Geometry check sheet. Reference: the model listing, model coordinates, mm. Round coordinates to 2 decimals unless told otherwise and drop trailing zeros. Order: outer loops, then holes, each group sorted by start corner. A loop starts at its lowest first (then second) coordinate and runs counter-clockwise, first axis right, second up. Notation, with made-up numbers: (-10, -23) -> (5, -23) arc R30 cw to (5, 2) -> close; hole circle Ø7 at (65.25, -25.5). An arc over 180 degrees is marked (long way). Use a Markdown table: item, result. Add a question column.
Item 1: Gauge pin test, flat ends, axial feed: pin 1 Ø4.5 at (y, z) = (8, 2.23) entering from -X; pin 2 Ø6 at (y, z) = (8, 2.23) entering from -X. Record the tip position at first contact, or that the pin passes through.
Item 2: Sectioned sample at B-B, the plane y = 284.5. Record the cut outline in (x, z), and give its area (3 significant figures).
Item 3: Material ranges on probe 1 along X at (y, z) = (335.5, 6.75); probe 2 along Z at (x, y) = (3, 106); probe 3 along Y at (x, z) = (9, 2), recorded low to high. Write a range as [from, to].
Item 4: Sectioned sample at A-A, the plane x = 0.25. Record the cut outline in (y, z).
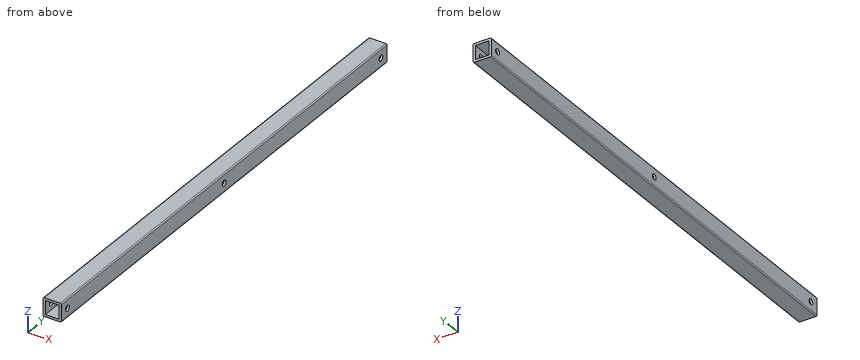
from build123d import *

# Parameters (mm, degrees)
SKETCH1_W           = 16
SKETCH1_H           = 16
SKETCH1_W_2         = 12
SKETCH1_H_2         = 12
BOSS_EXTRUDE1_DEPTH = 432
FILLET1_R           = 1
SKETCH2_R           = 2.5
CUT_EXTRUDE1_DEPTH  = 16
SKETCH3_R           = 2.5
CUT_EXTRUDE2_DEPTH  = 16


with BuildPart() as part:
    # Sketch1 → Boss-Extrude1 (new body)
    with BuildSketch(Plane(origin=(0, 0, 0), x_dir=(1, 0, 0), z_dir=(0, 1, 0))):
        with Locations((2.483870968, -2.225806452)):
            Rectangle(SKETCH1_W, SKETCH1_H)
        with Locations((2.483870968, -2.225806452)):
            Rectangle(SKETCH1_W_2, SKETCH1_H_2, mode=Mode.SUBTRACT)
    extrude(amount=BOSS_EXTRUDE1_DEPTH)

    # Fillet1
    fillet1_edges = [part.edges().sort_by_distance(p)[0] for p in [
        (-5.516129032, 216, -5.774193548),
        (10.483870968, 216, -5.774193548),
        (10.483870968, 216, 10.225806452),
        (-5.516129032, 216, 10.225806452),
    ]]
    fillet(fillet1_edges, radius=FILLET1_R)

    # Sketch2 → Cut-Extrude1 (cut)
    with BuildSketch(Plane.ZY.offset(5.516129032)):
        with Locations((2.225806452, 424)):
            Circle(SKETCH2_R)
        with Locations((2.225806452, 8)):
            Circle(SKETCH2_R)
    extrude(amount=-CUT_EXTRUDE1_DEPTH, mode=Mode.SUBTRACT)

    # Sketch3 → Cut-Extrude2 (cut)
    with BuildSketch(Plane.ZY.offset(5.516129032)):
        with Locations((2.225806452, 216)):
            Circle(SKETCH3_R)
    extrude(amount=-CUT_EXTRUDE2_DEPTH, mode=Mode.SUBTRACT)


solid = part.part
Found:
| question | item | result |
|---|---|---|
| 1 | pin 1 | passes through |
| 1 | pin 2 | stops at x = -5.52 |
| 2 | outline | (-5.52, -4.77) arc R1 ccw to (-4.52, -5.77) -> (9.48, -5.77) arc R1 ccw to (10.48, -4.77) -> (10.48, 9.23) arc R1 ccw to (9.48, 10.23) -> (-4.52, 10.23) arc R1 ccw to (-5.52, 9.23) -> close; hole (-3.52, -3.77) -> (8.48, -3.77) -> (8.48, 8.23) -> (-3.52, 8.23) -> close |
| 2 | area | 111 mm2 |
| 3 | probe 1 | x = [-5.52, -3.52], [8.48, 10.48] |
| 3 | probe 2 | z = [-5.77, -3.77], [8.23, 10.23] |
| 3 | probe 3 | y = [0, 5.51], [10.49, 213.51], [218.49, 421.51], [426.49, 432] |
| 4 | outline | (0, -5.77) -> (432, -5.77) -> (432, -3.77) -> (0, -3.77) -> close; (0, 8.23) -> (432, 8.23) -> (432, 10.23) -> (0, 10.23) -> close |
